CAD build for the part. Positions are in the model's coordinates, mm. A direction names the side the tool comes from. Round coordinates to 2 decimals unless told otherwise and drop trailing zeros. Order: outer loops, then holes, each group sorted by start corner. A loop starts at its lowest first (then second) coordinate and runs counter-clockwise, first axis right, second up. Notation, with made-up numbers: (-10, -20) -> (30, -20) arc R18 ccw to (30, 1) -> close; hole circle Ø2 at (78.5, 32). An arc over 180 degrees is marked (long way). Return JSON: item names as keys, results as strings. Group by question number.
Q1. Cut at A-A (y = 42.15). Write the cut outline in (x, z).
Q2. Cut at B-B (x = 5.75). Write the cut outline in (y, z).
Q3. Cut at D-D (z = 0.85). Write the cut outline in (x, y), then the cut area to 3 significant figures.
Q4. Flat gauge pins, fed straight in: pin 1 (2.5 mm diameter, centred on x = -7, y = 42, fed in from -Z); pin 2 (1.5 mm diameter, centred on x = -4, z = 1, fed in from -Y); pin 3 (3 mm diameter, centred on x = 3.5, z = -0.5, fed in from -Y). Where does each tip first touch, or does it go through?
Q5. Probe line 1 along X through (y, z) = (41.25, -1.7); line 2 along Z through (x, y) = (-7.5, 41.5); line 3 along X through (y, z) = (43.5, -1). List the from-to ranges inside material, lowest first.
Q6. Cut at C-C (z = -2.45). Write the cut outline in (x, y).
Q7. Which spindle directions (+Z, -Z, +X, -X, +Y, -Y) get a long thin tool onto all of the face, cutting with end or side? Do faces 1 (the flat face through (6, 44, -1.8)), 2 (the flat face through (6, 44, -1.4)), 3 (the flat face through (-6, 42, -1.8)), 4 (the flat face through (-1, 46, -0.4)), 5 (the flat face through (-6, 42, -1.4)). Say none if no direction does.
from build123d import *

# Parameters (mm, degrees)
REVOLUTION005_ANGLE     = -180
PAD023_DEPTH            = 0.4
BODY024_PLACEMENT_ANGLE = 180
PAD022_DEPTH            = 2.4


with BuildPart() as light005:
    # Sketch036 (on Face1 of ShapeBinder011) → Revolution005 (revolve)
    with BuildSketch(Plane.XY.offset(2.4)):
        with BuildLine():
            ThreePointArc((-2.75, 0), (0, -2.75), (2.75, 0))
            Line((-2.75, 0), (2.75, 0))
        make_face()
    revolve(axis=Axis((-2.75, 0, 2.4), (1, 0, 0)), revolution_arc=REVOLUTION005_ANGLE)


with BuildPart() as body024:
    # Sketch037 (on Face1 of ShapeBinder012) → Pad023 (new body)
    with BuildSketch(Plane(origin=(0, 0, 0), x_dir=(1, 0, 0), z_dir=(0, 0, -1))):
        with BuildLine():
            Line((3.65, 1.5), (6.65, 1.5))
            Line((6.65, 1.5), (6.65, 2))
            Line((6.65, 2), (8.65, 2))
            Line((8.65, 2), (8.65, 0.2))
            Line((8.65, 0.2), (6.65, 0.2))
            Line((6.65, 0.2), (6.65, 0.7))
            Line((6.65, 0.7), (4.45, 0.7))
            Line((4.45, 0.7), (4.45, -0.2))
            ThreePointArc((4.45, -0.2), (3.8, -0.85), (4.45, -1.5))
            Line((4.45, -1.5), (-6.65, -1.5))
            Line((-6.65, -1.5), (-6.65, -1.85))
            Line((-6.65, -1.85), (-8.65, -1.85))
            Line((-8.65, -1.85), (-8.65, -0.25))
            Line((-8.65, -0.25), (-6.65, -0.25))
            Line((-6.65, -0.25), (-6.65, -0.6))
            Line((-6.65, -0.6), (-4.95, -0.6))
            Line((-4.95, -0.6), (-4.95, 1.5))
            Line((-4.95, 1.5), (3.65, 1.5))
        make_face()
    extrude(amount=-PAD023_DEPTH)


with BuildPart() as body024_1:
    # Body024 placement: moved
    add(body024.part.moved(Location((0, 0, 1.4))).rotate(Axis((0, 0, 1.4), (1, 0, 0)), BODY024_PLACEMENT_ANGLE))


with BuildPart() as led6:
    # Sketch035 → Pad022 (new body)
    with BuildSketch(Plane.XY):
        with BuildLine():
            Line((-3.65, 1.75), (-3.65, -1.75))
            ThreePointArc((-3.65, -1.75), (0, -4), (3.65, -1.75))
            Line((3.65, 1.75), (3.65, -1.75))
            ThreePointArc((3.65, 1.75), (0, 4), (-3.65, 1.75))
        make_face()
    extrude(amount=PAD022_DEPTH)

    # Fusion006: union light005, Body024
    add(light005.part)
    add(body024_1.part)


with BuildPart() as led6_1:
    # Fusion006 placement: moved
    add(led6.part.moved(Location((0, 43, -2.8))))


solid = led6_1.part
Solution:
{
 "1": {"outline": "(-8.65, -1.8) -> (-3.65, -1.8) -> (-3.65, -2.8) -> (3.65, -2.8) -> (3.65, -1.8) -> (3.8, -1.8) -> (3.8, -1.4) -> (3.65, -1.4) -> (3.65, -0.4) -> (2.62, -0.4) arc R2.62 ccw to (-2.62, -0.4) -> (-3.65, -0.4) -> (-3.65, -1.4) -> (-8.65, -1.4) -> close"},
 "2": {"outline": "(43.7, -1.8) -> (44.5, -1.8) -> (44.5, -1.4) -> (43.7, -1.4) -> close"},
 "3": {"outline": "circle Ø4.9 at (0, 43)", "area": "18.8 mm²"},
 "4": {"pin 1": "stops at z = -1.8", "pin 2": "passes through", "pin 3": "stops at y = 39.52"},
 "5": {"line 1": "x = -8.65 to -6.65, -3.65 to 3.65", "line 2": "z = -1.8 to -1.4", "line 3": "x = -3.65 to 3.65"},
 "6": {"outline": "(-3.65, 41.25) arc R4.09 ccw to (3.65, 41.25) -> (3.65, 44.75) arc R4.09 ccw to (-3.65, 44.75) -> close"},
 "7": {"face 1": "-Z, +X, +Y, -Y", "face 2": "+Z, +X, +Y, -Y", "face 3": "-Z, -X, +Y, -Y", "face 4": "+Z", "face 5": "+Z, -X, +Y, -Y"}
}
